Check sheet for the modelled part. Datum: model origin and axes. Units: mm. A direction names the side the tool comes from. Round coordinates to 2 decimals unless told otherwise and drop trailing zeros. Write each loop counter-clockwise with the first axis right and the second up, starting at its lowest first coordinate (ties: lowest second). Pieces come first, ordered by that corner, then holes.
Item 1: Set-up check for faces 1 (the flat face through (9.14, -6.31, 1.48)), 2 (the flat face through (-45, 0, 1)), 3 (the flat face through (45, 0, 1)), 4 (the flat face through (1, 31, 1)), 5 (the flat face through (-1, -31, 1)): record each of +Z, -Z, +X, -X, +Y, -Y from which the full face is reachable in a straight line by a thin tool's end or side.
Item 2: Material ranges on line 1 along Y through (x, z) = (-20, 0.8); line 2 along Y through (x, z) = (-12.5, 0.1); line 3 along X through (y, z) = (6, 2.45), recorded low to high.
Item 3: Section check B-B, the plane x = -5. Record the cut outline in (y, z).
Item 4: Section check A-A, the plane y = -24.5. Record the cut outline in (x, z).
Item 5: Depth check by flat-ended pin: pin 1 (1.3 mm diameter, centred on x = -19, y = 24.5, fed in from +Z); pin 2 (0.9 mm diameter, centred on y = 3, z = 2, fed in from +X); pin 3 (0.9 mm diameter, centred on x = -13.5, z = 1.5, fed in from -Y). Enter the tip coordinate at first touch or a pass-through.
Item 6: Section check C-C, the plane y = 0. Record the cut outline in (x, z), plus the area to 3 significant figures.
Item 7: Section check D-D, the plane x = -19. Record the cut outline in (y, z), plus the area to 3 significant figures.
from build123d import *

# Parameters (mm, degrees)
F1_DEPTH = 3
F2_R     = 5
F4_D     = 2.2


with BuildPart() as f1:
    # F0 (on Top) → F1 (new body)
    with BuildSketch(Plane.XY):
        with BuildLine():
            ThreePointArc((-45, -26), (-48.5355339059, -34.5355339059), (-40, -31))
            Line((-40, -31), (-43.5, -31))
            ThreePointArc((-43.5, -31), (-46.0606601718, -32.0606601718), (-45, -29.5))
            Line((-45, -29.5), (-45, -26))
        make_face()
        with BuildLine():
            ThreePointArc((-45, -26), (-41.4644660941, -27.4644660941), (-40, -31))
            Line((-40, -31), (40, -31))
            ThreePointArc((40, -31), (41.4644660941, -27.4644660941), (45, -26))
            Line((45, -26), (45, 26))
            ThreePointArc((45, 26), (41.4644660941, 27.4644660941), (40, 31))
            Line((40, 31), (-40, 31))
            ThreePointArc((-40, 31), (-41.4644660941, 27.4644660941), (-45, 26))
            Line((-45, 26), (-45, -26))
        make_face()
        with BuildLine():
            Line((-11.0606601718, -8.9393398282), (8.9393398282, 11.0606601718))
            ThreePointArc((8.9393398282, 11.0606601718), (36.4956890143, -0.3535533906), (8.9393398282, -11.767766953))
            Line((8.9393398282, -11.767766953), (3.7625631329, -6.5909902577))
            Line((3.7625631329, -6.5909902577), (5.1767766953, -5.1767766953))
            Line((5.1767766953, -5.1767766953), (6.5909902577, -3.7625631329))
            Line((6.5909902577, -3.7625631329), (11.767766953, -8.9393398282))
            ThreePointArc((11.767766953, -8.9393398282), (32.4956890143, -0.3535533906), (11.767766953, 8.232233047))
            Line((11.767766953, 8.232233047), (-8.232233047, -11.767766953))
            ThreePointArc((-8.232233047, -11.767766953), (-36.6421356237, 0), (-8.232233047, 11.767766953))
            ThreePointArc((-8.232233047, 11.767766953), (-8.2074655375, 11.7425578811), (-8.1831473235, 11.716915118))
            Line((-8.1831473235, 11.716915118), (-3.3599240188, 6.5401384227))
            Line((-3.3599240188, 6.5401384227), (-4.8232233047, 5.1767766953))
            Line((-4.8232233047, 5.1767766953), (-6.2865225906, 3.8134149679))
            Line((-6.2865225906, 3.8134149679), (-11.0847678218, 8.9633826393))
            ThreePointArc((-11.0847678218, 8.9633826393), (-32.6421241617, -0.0170237742), (-11.0606601718, -8.9393398282))
        make_face(mode=Mode.SUBTRACT)
        with BuildLine():
            Line((-43.5, -31), (-40, -31))
            ThreePointArc((-40, -31), (-41.4644660941, -27.4644660941), (-45, -26))
            Line((-45, -26), (-45, -29.5))
            ThreePointArc((-45, -29.5), (-43.9393398282, -29.9393398282), (-43.5, -31))
        make_face()
        with BuildLine():
            ThreePointArc((45, -26), (41.4644660941, -27.4644660941), (40, -31))
            Line((40, -31), (43.5, -31))
            ThreePointArc((43.5, -31), (43.9393398282, -29.9393398282), (45, -29.5))
            Line((45, -29.5), (45, -26))
        make_face()
        with BuildLine():
            Line((43.5, -31), (40, -31))
            ThreePointArc((40, -31), (45, -36), (50, -31))
            ThreePointArc((50, -31), (48.5355339059, -27.4644660941), (45, -26))
            Line((45, -26), (45, -29.5))
            ThreePointArc((45, -29.5), (46.0606601718, -29.9393398282), (46.5, -31))
            ThreePointArc((46.5, -31), (45, -32.5), (43.5, -31))
        make_face()
        with BuildLine():
            ThreePointArc((-40, 31), (-48.5355339059, 34.5355339059), (-45, 26))
            Line((-45, 26), (-45, 29.5))
            ThreePointArc((-45, 29.5), (-46.0606601718, 32.0606601718), (-43.5, 31))
            Line((-43.5, 31), (-40, 31))
        make_face()
        with BuildLine():
            Line((-45, 29.5), (-45, 26))
            ThreePointArc((-45, 26), (-41.4644660941, 27.4644660941), (-40, 31))
            Line((-40, 31), (-43.5, 31))
            ThreePointArc((-43.5, 31), (-43.9393398282, 29.9393398282), (-45, 29.5))
        make_face()
        with BuildLine():
            ThreePointArc((40, 31), (41.4644660941, 27.4644660941), (45, 26))
            Line((45, 26), (45, 29.5))
            ThreePointArc((45, 29.5), (43.9393398282, 29.9393398282), (43.5, 31))
            Line((43.5, 31), (40, 31))
        make_face()
        with BuildLine():
            Line((45, 29.5), (45, 26))
            ThreePointArc((45, 26), (48.5355339059, 27.4644660941), (50, 31))
            ThreePointArc((50, 31), (45, 36), (40, 31))
            Line((40, 31), (43.5, 31))
            ThreePointArc((43.5, 31), (45, 32.5), (46.5, 31))
            ThreePointArc((46.5, 31), (46.0606601718, 29.9393398282), (45, 29.5))
        make_face()
    extrude(amount=F1_DEPTH)

    # F2
    f2_edges = [f1.edges().sort_by_distance(p)[0] for p in [
        (-40, -31, 1.5),
        (45, 26, 1.5),
        (40, -31, 1.5),
        (-45, -26, 1.5),
        (-45, 26, 1.5),
        (-40, 31, 1.5),
        (40, 31, 1.5),
        (45, -26, 1.5),
    ]]
    fillet(f2_edges, radius=F2_R)

    # F4 (through all)
    with Locations(Plane.XY.offset(3)):
        with Locations((-19, 24.5), (39, 24.5), (39, -24.5), (-19, -24.5)):
            Hole(F4_D / 2)


solid = f1.part
Values found:
1. face 1: +Z, -Z
1. face 2: +Z, -Z, -X
1. face 3: +Z, -Z, +X
1. face 4: +Z, -Z, +Y
1. face 5: +Z, -Z, -Y
2. line 1: y = -31 to -24.96, -24.04 to -16.64, -12.64 to 12.64, 16.64 to 24.04, 24.96 to 31
2. line 2: y = -31 to -14.86, -10.18 to 10.18, 14.86 to 31
2. line 3: x = -45 to -35.52, -31.13 to -8.32, -3.94 to 3.88, 9.54 to 30.7, 35.19 to 45
3. outline: (-31, 0) - (-8.54, 0) - (-8.54, 3) - (-31, 3) - close; (-2.88, 0) - (5.01, 0) - (5.01, 3) - (-2.88, 3) - close; (8.3, 0) - (31, 0) - (31, 3) - (8.3, 3) - close
4. outline: (-45.49, 0) - (-20.1, 0) - (-20.1, 3) - (-45.49, 3) - close; (-17.9, 0) - (37.9, 0) - (37.9, 3) - (-17.9, 3) - close; (40.1, 0) - (45.49, 0) - (45.49, 3) - (40.1, 3) - close
5. pin 1: passes through
5. pin 2: stops at x = 45
5. pin 3: stops at y = -31
6. outline: (-45, 0) - (-36.64, 0) - (-36.64, 3) - (-45, 3) - close; (-32.64, 0) - (-2.12, 0) - (-2.12, 3) - (-32.64, 3) - close; (3.54, 0) - (32.49, 0) - (32.49, 3) - (3.54, 3) - close; (36.49, 0) - (45, 0) - (45, 3) - (36.49, 3) - close
6. area: 229 mm2
7. outline: (-31, 0) - (-25.6, 0) - (-25.6, 3) - (-31, 3) - close; (-23.4, 0) - (-16.61, 0) - (-16.61, 3) - (-23.4, 3) - close; (-12.6, 0) - (12.6, 0) - (12.6, 3) - (-12.6, 3) - close; (16.61, 0) - (23.4, 0) - (23.4, 3) - (16.61, 3) - close; (25.6, 0) - (31, 0) - (31, 3) - (25.6, 3) - close
7. area: 149 mm2
